For this review, take the finished solid that the model builds, in its own axes (mm). Face numbers are marked on the shaded views. A direction names the side the tool comes from. Round coordinates to 2 decimals unless told otherwise and drop trailing zeros. Order: outer loops, then holes, each group sorted by start corner. A loop starts at its lowest first (then second) coordinate and runs counter-clockwise, first axis right, second up. Notation, with made-up numbers: (-5, 76) -> (43, 76) arc R18 cw to (43, 81) -> close; hole circle Ø10 at (-9, -33.5). An arc over 180 degrees is marked (long way). Use a Markdown table: item, result. Add a question column.
1) Consider section B-B (x = 0.4). State the section outline as (y, z) points.
2) Consider section A-A (x = 2.35). State the section outline as (y, z) points.
3) Wall thickness on line 1 along X through (y, z) = (44, 17.25); line 2 along Z through (x, y) = (0.95, 44.75); line 3 along Y through (x, z) = (0.95, 18.5): over which ranges is each line inside the solid? List them lowest first. Write a range as [from, to].
4) Clearance check with flat-ended pins moving along their axes: P1, Ø2, axis at x = 3.5, y = 37, coming from the -Z side; P2, Ø1, axis at x = 3.5, z = 25, coming from the -Y side; P3, Ø0.9, axis at y = 36.1, z = 19.32, coming from the +X side. State where each tip first meets the part, or that it passes through.
5) Machinability: for the marked faces 1 and 2, which of the approach directions +Z, -Z, +X, -X, +Y, -Y give a long, thin tool a straight path to every point of the face, cutting with its end or side? Answer none if there is none.
```python
from build123d import *

# Parameters (mm, degrees)
F0_R     = 10
F1_DEPTH = 2
F2_R     = 1.5
F2_R_2   = 0.75
F3_DEPTH = 2
F4_R     = 0.99999


# Not quite as in the source:
# - a fillet or chamfer is up to 0.001 mm smaller than in the source, because OpenCascade refuses the exact size


with BuildPart() as f1:
    # F0 (on Right) → F1 (new body)
    with BuildSketch(Plane.YZ):
        with Locations((36.0975265503, 19.3211734295)):
            Circle(F0_R)
    extrude(amount=F1_DEPTH)

    # F2 (on face) → F3 (join)
    with BuildSketch(Plane.YZ.offset(2)):
        with Locations((36.0975265503, 19.3211734295)):
            Circle(F2_R)
        with Locations((36.0975265503, 19.3211734295)):
            Circle(F2_R_2, mode=Mode.SUBTRACT)
    extrude(amount=F3_DEPTH)

    # F4 (radius 1 in the source; OpenCascade refuses exactly that, so slightly less here)
    f4_edges = [f1.edges().sort_by_distance(p)[0] for p in [
        (2, 26.097527, 19.321173),
        (0, 26.097527, 19.321173),
    ]]
    fillet(f4_edges, radius=F4_R)


solid = f1.part
```
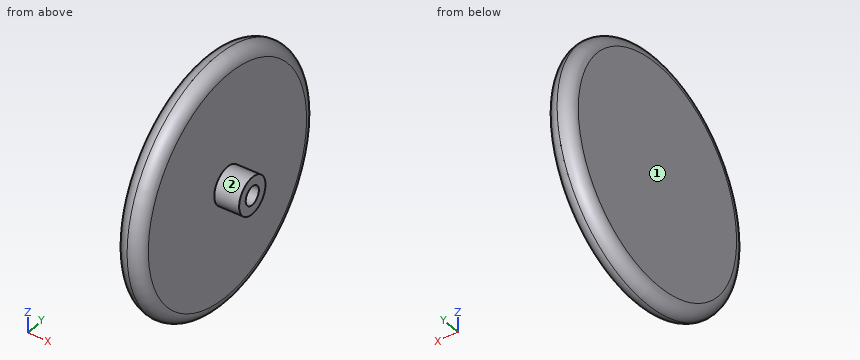
Results list:
| question | item | result |
|---|---|---|
| 1 | outline | circle Ø19.6 at (36.1, 19.32) |
| 2 | outline | circle Ø3 at (36.1, 19.32); hole circle Ø1.5 at (36.1, 19.32) |
| 3 | line 1 | [0, 2] |
| 3 | line 2 | [14.31, 24.33] |
| 3 | line 3 | [26.13, 46.06] |
| 4 | P1 | z = 17.82 |
| 4 | P2 | through |
| 4 | P3 | x = 2 |
| 5 | face 1 | +Z, -Z, -X, +Y, -Y |
| 5 | face 2 | +X |
